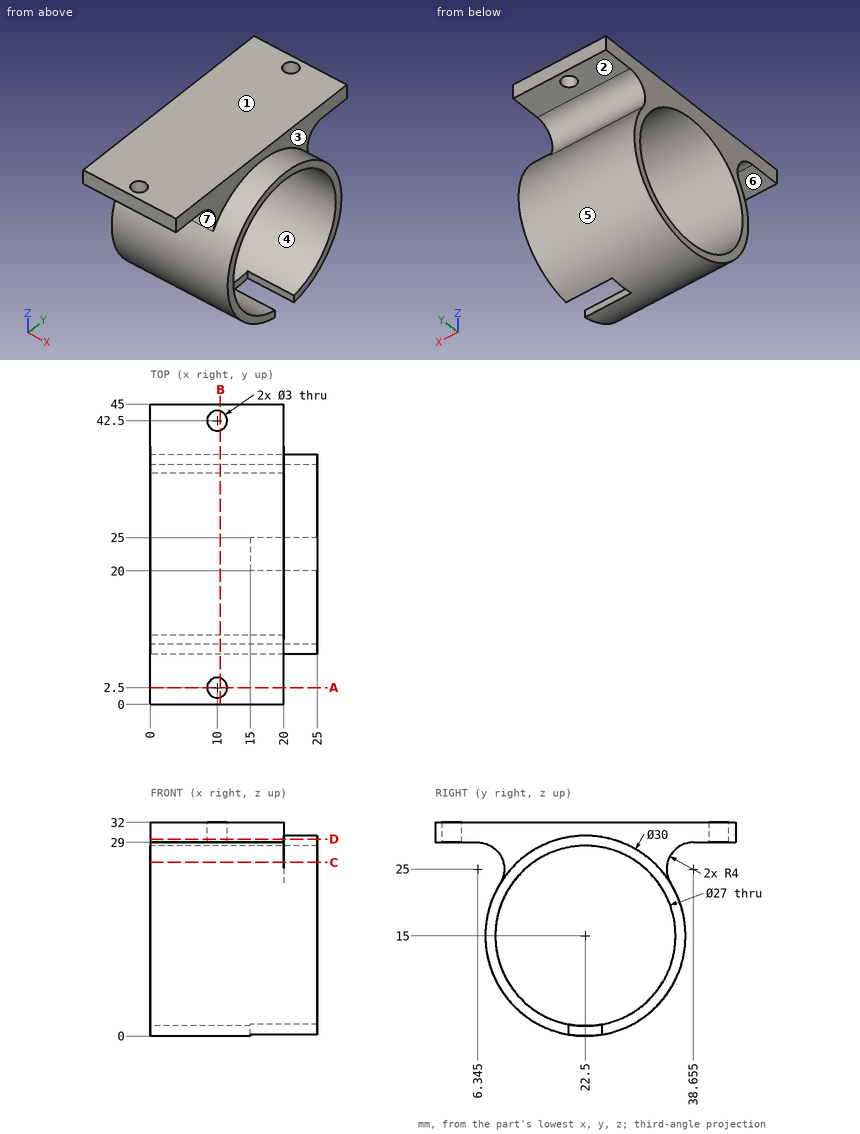
Design review of the part shown in the three views and the two pictorial views. Dimensions are in mm from the part's minimum x, y and z. A direction names the side the tool comes from. Round coordinates to 2 decimals unless told otherwise and drop trailing zeros. Order: outer loops, then holes, each group sorted by start corner. A loop starts at its lowest first (then second) coordinate and runs counter-clockwise, first axis right, second up.
Q1. We need section A-A, the plane y = 2.5. Give the boundary of the cut face in (x, z).
Findings below:
outline: (0, 29) - (8.5, 29) - (8.5, 32) - (0, 32) - close; (11.5, 29) - (20, 29) - (20, 32) - (11.5, 32) - close
Q2. We need section D-D, the plane z = 29.5. Give the boundary of the cut face in (x, y), plus the area to 3 significant figures.
Findings below:
outline: (0, 0) - (20, 0) - (20, 18.66) - (25, 18.66) - (25, 26.34) - (20, 26.34) - (20, 45) - (0, 45) - close; hole circle Ø3 at (10, 2.5); hole circle Ø3 at (10, 42.5)
area: 924 mm2
Q3. Insertion check: P1, Ø2, axis at x = 16, z = 13.5, coming from the -Y side; P2, Ø1.2, axis at x = 18, z = 1, coming from the -Y side; P3, Ø1.2, axis at x = 18, z = 0.5, coming from the +Y side (1 decimal); P4, Ø5, axis at y = 12, z = 13, coming from the -X side. Each pin has a flat end and moves straight along its axis. Give the tip position at first contact, or say it passes through.
Findings below:
P1: stops at y = 7.51
P2: stops at y = 15.76
P3: stops at y = 28.1
P4: passes through
Q4. Mouldability with a two-part tool opening along Y and no side actions: class the marked faces 4, 5, 6 and 7 as pulls with the +Y half, pulls with the -Y half, needs draft (parallel to the pull), parting line crosses it, or undercut.
Findings below:
face 4: undercut
face 5: parting line crosses it
face 6: needs draft
face 7: pulls with the -Y half
Q5. Wall thickness on line 1 (Z direction, x = 9, y = 22); line 2 (X direction, y = 42.5, z = 29.7); line 3 (Y direction, x = 19.25, z = 15): over which ranges is each line inside the solid? List them lowest first.
Findings below:
line 1: z = 0.01 to 1.51, 28.49 to 32
line 2: x = 0 to 8.5, 11.5 to 20
line 3: y = 7.5 to 9, 36 to 37.5
Q6. We need section C-C, the plane z = 26. Give the boundary of the cut face in (x, y), plus the area to 3 significant figures.
Findings below:
outline: (0, 10.22) - (20, 10.22) - (20, 12.3) - (25, 12.3) - (25, 14.67) - (0, 14.67) - close; (0, 30.33) - (25, 30.33) - (25, 32.7) - (20, 32.7) - (20, 34.78) - (0, 34.78) - close
area: 202 mm2
Q7. We need section B-B, the plane x = 10.5. Give the boundary of the cut face in (y, z) (1 decimal).
Findings below:
outline: (0, 29) - (1.1, 29) - (1.1, 32) - (0, 32) - close; (3.9, 29) - (6.3, 29) arc R4 cw to (9.7, 22.9) arc R15 ccw (long way) to (35.3, 22.9) arc R4 cw to (38.7, 29) - (41.1, 29) - (41.1, 32) - (3.9, 32) - close; (43.9, 29) - (45, 29) - (45, 32) - (43.9, 32) - close; hole circle Ø27 at (22.5, 15)
Q8. Machinability: for the marked faces 1, 2 and 3, which of the approach directions +Z, -Z, +X, -X, +Y, -Y give a long, thin tool a straight path to every point of the face, cutting with its end or side? Answer none if there is none.
Findings below:
face 1: +Z, +X, -X, +Y, -Y
face 2: -Z, +X, -X, +Y
face 3: +Z, +X
